Source: CAD feature listing. Evaluate the final solid. Frame: model axes, mm. A direction names the side the tool comes from. Round coordinates to 2 decimals unless told otherwise and drop trailing zeros. Loops run counter-clockwise (first coordinate to the right, second up) from the corner with the lowest first, then second, coordinate; pieces in that order, holes last. Notation, with made-up numbers: (57.25, 64) - (84.25, 64) arc R20 ccw to (84.25, 69) - close; hole circle Ø8 at (-27.5, 58). An arc over 180 degrees is marked (long way). One line per question, with ' | ' between items. Start each with the question number.
1. Cut plane D-D (y = -53). Return loops of the section in (x, z).
2. Cut plane A-A (x = 0). Return loops of the section in (y, z).
3. Mould query, pull axis Z, two halves, no side actions, for faces 3 (the flat face through (20, -76.2, 1)), 4 (the cylindrical face through (18.413, -111.262, 5.799)), 5 (the flat face through (0, -25.4, 0)). Classes: pulls with the +Z half, pulls with the -Z half, needs draft (parallel to the pull), parting line crosses it, or undercut.
4. Cut plane B-B (z = 0). Return loops of the section in (x, y).
5. Cut plane C-C (y = -119.5). Return loops of the section in (x, z), then the cut area to 3 significant figures.
6. Ray query, line 1 (Z direction, x = 0, y = -102); line 2 (Y direction, x = -7.5, z = -23); line 3 (Y direction, x = 7, z = -5.5). Return the intervals inside material, ascending.
7. Access query for faces 1 (the cylindrical face through (6.061, -89.789, 9.507)), 2 (the flat face through (-4, -152.4, 11)). Directions: +Z, -Z, +X, -X, +Y, -Y. A direction counts if a zero-diameter tool reaches every point of the face in a straight line with its end or side. Return the directions, or none.
8. Pin query (flat end, axial travel): pin 1 (6 mm diameter, centred on x = 39, y = -43, fed in from +Z); pin 2 (4 mm diameter, centred on x = 1.5, y = -102.5, fed in from -Z); pin 3 (5 mm diameter, centred on y = -58.5, z = -42.5, fed in from -X). Return the tip coordinate at first contact, or that it passes through.
```python
from build123d import *

# Parameters (mm, degrees)
F0_R      = 58.7395
F2_DEPTH  = 76.2
F3_R      = 19.30494
F4_DEPTH  = 76.2
F6_R      = 9.692855
F7_DEPTH  = 76.2
F5_R      = 9.656386
F8_DEPTH  = 127
F9_R      = 11.274603
F10_DEPTH = 127
F11_R     = 5.08
F12_SIZE  = 12.7


with BuildPart() as f2:
    # F0 (on Front) → F2 (new body)
    with BuildSketch(Plane.XZ):
        Circle(F0_R)
    extrude(amount=F2_DEPTH)

    # F3 (on face) → F4 (join)
    with BuildSketch(Plane.XZ.offset(76.2)):
        Circle(F3_R)
    extrude(amount=F4_DEPTH)

    # F6 (on Front) → F7 (cut)
    with BuildSketch(Plane.XZ):
        Circle(F6_R)
    extrude(amount=-F7_DEPTH, mode=Mode.SUBTRACT)

    # F5 (on Front) → F8 (cut)
    with BuildSketch(Plane.XZ):
        Circle(F5_R)
    extrude(amount=-F8_DEPTH, mode=Mode.SUBTRACT)

    # F9 (on face) → F10 (cut)
    with BuildSketch(Plane.XZ.offset(152.4)):
        Circle(F9_R)
    extrude(amount=-F10_DEPTH, mode=Mode.SUBTRACT)

    # F11
    f11_edges = [f2.edges().sort_by_distance(p)[0] for p in [
        (-19.30494, -152.4, 0),
    ]]
    fillet(f11_edges, radius=F11_R)

    # F12
    f12_edges = [f2.edges().sort_by_distance(p)[0] for p in [
        (-58.7395, -76.2, 0),
    ]]
    chamfer(f12_edges, length=F12_SIZE)


solid = f2.part
```
Answers follow:
1) outline: circle Ø117.48 at (0, 0); hole circle Ø22.55 at (0, 0)
2) outline: (-152.4, -14.22) arc R5.08 ccw to (-147.32, -19.3) - (-76.2, -19.3) - (-76.2, -46.04) - (-63.5, -58.74) - (0, -58.74) - (0, 58.74) - (-63.5, 58.74) - (-76.2, 46.04) - (-76.2, 19.3) - (-147.32, 19.3) arc R5.08 ccw to (-152.4, 14.22) - (-152.4, 11.27) - (-25.4, 11.27) - (-25.4, -11.27) - (-152.4, -11.27) - close
3) face 3: needs draft | face 4: parting line crosses it | face 5: undercut
4) outline: (-58.74, -63.5) - (-46.04, -76.2) - (-19.3, -76.2) - (-19.3, -147.32) arc R5.08 ccw to (-14.22, -152.4) - (-11.27, -152.4) - (-11.27, -25.4) - (11.27, -25.4) - (11.27, -152.4) - (14.22, -152.4) arc R5.08 ccw to (19.3, -147.32) - (19.3, -76.2) - (46.04, -76.2) - (58.74, -63.5) - (58.74, 0) - (-58.74, 0) - close
5) outline: circle Ø38.61 at (0, 0); hole circle Ø22.55 at (0, 0) | area: 771 mm2
6) line 1: z = -19.3 to -11.27, 11.27 to 19.3 | line 2: y = -76.2 to 0 | line 3: y = -25.4 to 0
7) face 1: -Y | face 2: +Z, -Z, +X, -X, -Y
8) pin 1: stops at z = 46.41 | pin 2: stops at z = -19.3 | pin 3: stops at x = -43.02
